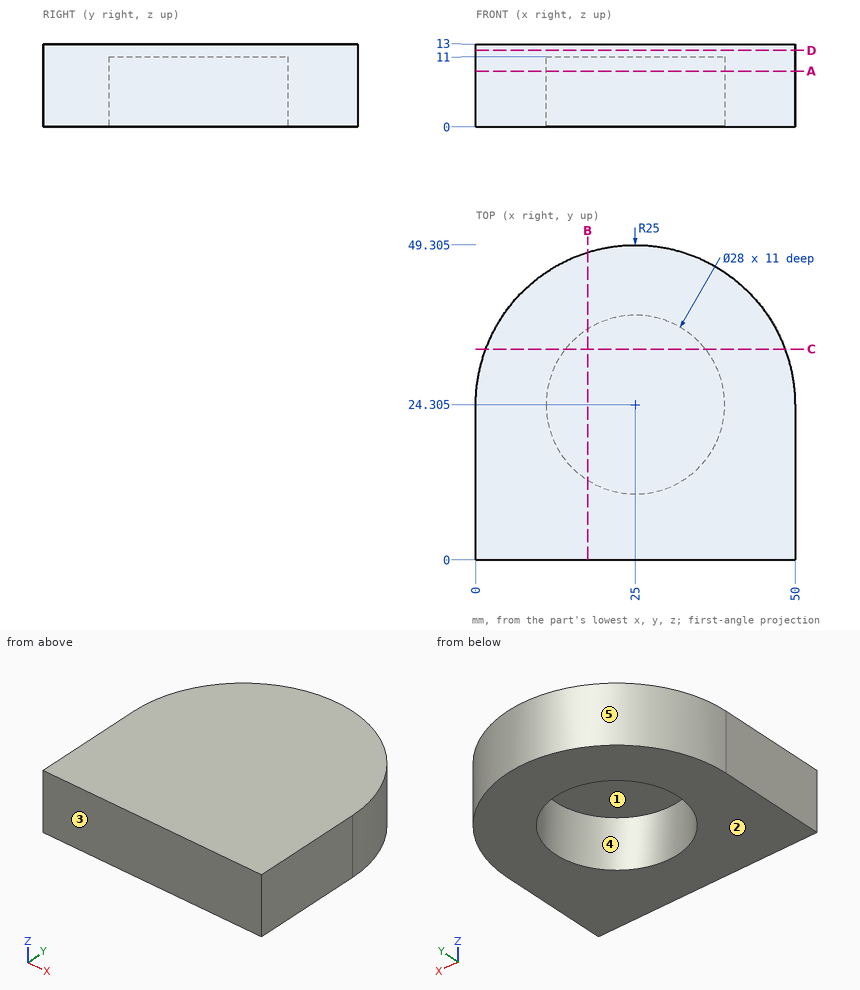
Input: dimensioned drawing with shaded views. Units: mm. Origin: part minimum x, y, z. A direction names the side the tool comes from. Round coordinates to 2 decimals unless told otherwise and drop trailing zeros. Write each loop counter-clockwise with the first axis right and the second up, starting at its lowest first coordinate (ties: lowest second). Pieces come first, ordered by that corner, then holes. Notation, with made-up numbers: (10.25, 6) -> (57.25, 6) arc R28 cw to (57.25, 44) -> close; hole circle Ø1 at (45.5, 79). An arc over 180 degrees is marked (long way). Use CSV: the item, a comma, the result in double quotes. Start each with the question number.
Q1. Pull-direction query (Y, two-part tool) for the marked faces 3, 4 and 5; classes: pulls with the +Y half, pulls with the -Y half, needs draft (parallel to the pull), parting line crosses it, or undercut.
Q2. Section D-D (z = 12). Return loops of the section in (x, y) (1 decimal).
Q3. Reachability of the marked faces 1 and 2 from +Z, -Z, +X, -X, +Y, -Y: full face, straight path, thin tool, end or side. Return the list, or none.
Q4. Line query: L1, parallel to Y at x = 25, z = 3.25 (1 decimal); L2, parallel to Y at x = 22.5, z = 6.5; L3, parallel to X at y = 28, z = 0.5 (1 decimal). Output: solid intervals per line, ascending.
Q5. Section A-A (z = 8.75). Return loops of the section in (x, y) (1 decimal).
Q6. First-contact query: pin 1 Ø2 at (y, z) = (30, 7.5) entering from +X (1 decimal); pin 2 Ø5 at (y, z) = (39.5, 5.5) entering from -X; pin 3 Ø2 at (y, z) = (35.5, 9.5) entering from -X. Flat tips, straight axial feed; report the tip coordinate or a pass-through.
Q7. Section C-C (y = 33). Return loops of the section in (x, z).
Q8. Section B-B (x = 17.5). Return loops of the section in (y, z).
Result sheet:
1,face 3,"pulls with the -Y half"
1,face 4,"undercut"
1,face 5,"pulls with the +Y half"
2,outline,"(0, 0) -> (50, 0) -> (50, 24.3) arc R25 ccw to (0, 24.3) -> close"
3,face 1,"-Z"
3,face 2,"-Z, +X, -X, +Y, -Y"
4,L1,"0 to 10.3, 38.3 to 49.3"
4,L2,"0 to 10.53, 38.08 to 49.18"
4,L3,"0.3 to 11.5, 38.5 to 49.7"
5,outline,"(0, 0) -> (50, 0) -> (50, 24.3) arc R25 ccw to (0, 24.3) -> close; hole circle Ø28 at (25, 24.3)"
6,pin 1,"x = 49.6"
6,pin 2,"x = 3.46"
6,pin 3,"x = 2.17"
7,outline,"(1.56, 0) -> (14.03, 0) -> (14.03, 11) -> (35.97, 11) -> (35.97, 0) -> (48.44, 0) -> (48.44, 13) -> (1.56, 13) -> close"
8,outline,"(0, 0) -> (12.48, 0) -> (12.48, 11) -> (36.13, 11) -> (36.13, 0) -> (48.15, 0) -> (48.15, 13) -> (0, 13) -> close"
